from build123d import *

# Parameters (mm, degrees)
LINEAR_AUSTRAGEN_D_NN1_DEPTH = 30


with BuildPart() as part:
    # Skizze1 → Linear-Austragen-Dünn1 (new body)
    with BuildSketch(Plane.XZ):
        with BuildLine():
            Line((0, 75), (130, 75))
            ThreePointArc((130, 75), (144.142135624, 69.142135624), (150, 55))
            Line((150, 55), (150, -150))
            Line((150, -150), (150, -151))
            Line((150, -151), (151, -151))
            Line((151, -151), (151, -150))
            Line((151, -150), (151, 55))
            ThreePointArc((151, 55), (144.849242405, 69.849242405), (130, 76))
            Line((130, 76), (0, 76))
            Line((0, 76), (0, 75))
        make_face()
    linear_austragen_d_nn1 = extrude(amount=-LINEAR_AUSTRAGEN_D_NN1_DEPTH)

    # Spiegeln1: Linear-Austragen-Dünn1 across plane
    add(linear_austragen_d_nn1.mirror(Plane(origin=(0, 30, 75), x_dir=(0, 0, 1), z_dir=(1, 0, 0))))


solid = part.part
For this review, take the finished solid that the model builds, in its own axes (mm). A direction names the side the tool comes from. Coordinates: 2 decimals unless noted, no trailing zeros. Loops run counter-clockwise (first coordinate to the right, second up) from the corner with the lowest first, then second, coordinate; pieces in that order, holes last. Notation, with made-up numbers: (33.5, -12.75) - (91.5, -12.75) arc R22 cw to (91.5, 6.25) - close; hole circle Ø1 at (37, -13.5). An arc over 180 degrees is marked (long way). Return JSON: item names as keys, results as strings.
Item 1: Take a section at C-C (x = 23.5). Give the boundary of the cut face in (y, z).
Determined:
{"outline": "(0, 75) - (30, 75) - (30, 76) - (0, 76) - close"}
Item 2: Insertion check: pin 1 (2 mm diameter, centred on x = 24.5, y = 11, fed in from -Z). The pin has a flat end and moves straight along its axis. Give the tip position at first contact, or say it passes through.
Determined:
{"pin 1": "stops at z = 75"}
Item 3: Take a section at A-A (z = -109.5). Give the boundary of the cut face in (x, y), then the cut area to 3 significant figures.
Determined:
{"outline": "(-151, 0) - (-150, 0) - (-150, 30) - (-151, 30) - close; (150, 0) - (151, 0) - (151, 30) - (150, 30) - close", "area": "60.0 mm2"}
Item 4: For faces 5 (the cylindrical face through (-143.986, 14.79, 69.297)), 6 (the flat face through (151, 15, -49)), list the 3-axis set-ups (+Z, -Z, +X, -X, +Y, -Y) from which the entire face can be reached by the end or side of a thin tool; tool diameter is ignored.
Determined:
{"face 5": "-Z, +Y, -Y", "face 6": "+Z, -Z, +X, +Y, -Y"}
Item 5: Mouldability with a two-part tool opening along X and no side actions: class faces 1 (the cylindrical face through (145.012, 14.79, 69.685)), 2 (the cylindrical face through (143.986, 14.79, 69.297)), 3 (the flat face through (-2, 15, 76)), 4 (the cylindrical face through (-145.012, 14.79, 69.685)) as pulls with the +X half, pulls with the -X half, needs draft (parallel to the pull), parting line crosses it, or undercut.
Determined:
{"face 1": "pulls with the +X half", "face 2": "undercut", "face 3": "needs draft", "face 4": "pulls with the -X half"}
Item 6: For line 1 (X direction, y = 27, z = -11); line 2 (Z direction, x = 65, y = 9); line 3 (Z direction, x = -133.5, y = 20.25), list the stretches that pass through material, from the lowest coordinate up.
Determined:
{"line 1": "x = -151 to -150, 150 to 151", "line 2": "z = 75 to 76", "line 3": "z = 74.69 to 75.71"}
Item 7: Take a section at B-B (y = 17). Give the boundary of the cut face in (x, z).
Determined:
{"outline": "(-151, -151) - (-150, -151) - (-150, 55) arc R20 cw to (-130, 75) - (130, 75) arc R20 cw to (150, 55) - (150, -151) - (151, -151) - (151, 55) arc R21 ccw to (130, 76) - (-130, 76) arc R21 ccw to (-151, 55) - close"}
